```python
from build123d import *

# Parameters (mm, degrees)
SKETCH1_R           = 3.5
BOSS_EXTRUDE1_DEPTH = 2
SKETCH2_R           = 2.75
BOSS_EXTRUDE2_DEPTH = 50.5
SKETCH3_R           = 3.25
BOSS_EXTRUDE3_DEPTH = 1
FILLET1_R           = 1.5
FILLET2_R           = 0.35
FILLET3_R           = 0.2


with BuildPart() as part:
    # Sketch1 → Boss-Extrude1 (new body)
    with BuildSketch(Plane(origin=(0, 0, 0), x_dir=(0, 0, -1), z_dir=(1, 0, 0))):
        Circle(SKETCH1_R)
    extrude(amount=BOSS_EXTRUDE1_DEPTH)

    # Sketch2 → Boss-Extrude2 (add)
    with BuildSketch(Plane(origin=(2, 0, 0), x_dir=(0, 0, -1), z_dir=(1, 0, 0))):
        Circle(SKETCH2_R)
    extrude(amount=BOSS_EXTRUDE2_DEPTH)

    # Sketch3 → Boss-Extrude3 (add)
    with BuildSketch(Plane(origin=(52.5, 0, 0), x_dir=(0, 0, -1), z_dir=(1, 0, 0))):
        Circle(SKETCH3_R)
    extrude(amount=BOSS_EXTRUDE3_DEPTH)

    # Fillet1
    fillet1_edges = [part.edges().sort_by_distance(p)[0] for p in [
        (0, 0, 3.5),
    ]]
    fillet(fillet1_edges, radius=FILLET1_R)

    # Fillet2
    fillet2_edges = [part.edges().sort_by_distance(p)[0] for p in [
        (52.5, 0, 3.25),
    ]]
    fillet(fillet2_edges, radius=FILLET2_R)

    # Fillet3
    fillet3_edges = [part.edges().sort_by_distance(p)[0] for p in [
        (53.5, 0, 3.25),
    ]]
    fillet(fillet3_edges, radius=FILLET3_R)


solid = part.part
```
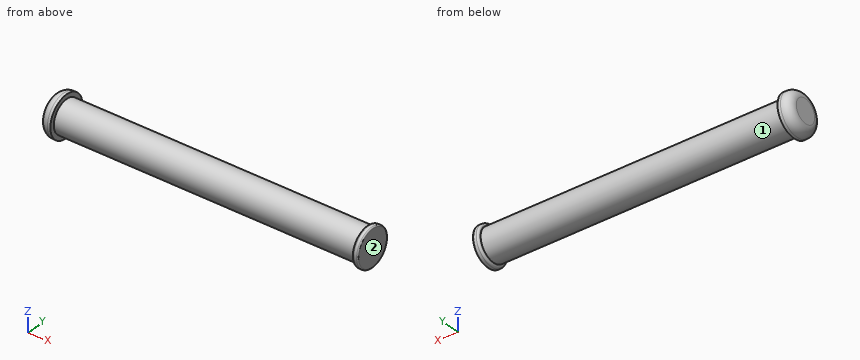
Geometry: final body of the model. Coordinates: model frame, mm. Face numbers are marked on the shaded views. Coordinates: 2 decimals unless noted, no trailing zeros. Order: outer loops, then holes, each group sorted by start corner. A loop starts at its lowest first (then second) coordinate and runs counter-clockwise, first axis right, second up.
Item 1: Draft query along X for the marked faces 1 and 2. Return one class per face: released by +X, released by -X, zero draft, split by the parting line, or undercut.
Answer:
face 1: undercut
face 2: released by +X
Item 2: Material intervals for line 1 along X through (y, z) = (-1.5, 1.5); line 2 along X through (y, z) = (-1, 3); line 3 along Z through (x, y) = (34, 0.25), sorted ascending.
Answer:
line 1: x = 0 to 53.5
line 2: x = 0.55 to 2, 52.62 to 53.47
line 3: z = -2.74 to 2.74
Item 3: Section query C-C (x = 47.5). Output: boundary loops of the cut face in (y, z), then the cut area to 3 significant figures.
Answer:
outline: circle Ø5.5 at (0, 0)
area: 23.8 mm2
Item 4: Contact query for flat-ended pins moving along their axis: P1, Ø4, axis at x = 31, y = 1, coming from the -Z side; P2, Ø1.5, axis at x = 44, z = -1.5, coming from the +Y side. Output: stop coordinate, or through.
Answer:
P1: stops at z = -2.75
P2: stops at y = 2.65
Item 5: Section query A-A (z = 0). Output: boundary loops of the cut face in (x, y), then the cut area to 3 significant figures.
Answer:
outline: (0, -2) arc R1.5 ccw to (1.5, -3.5) - (2, -3.5) - (2, -2.75) - (52.5, -2.75) - (52.5, -2.9) arc R0.35 ccw to (52.85, -3.25) - (53.3, -3.25) arc R0.2 ccw to (53.5, -3.05) - (53.5, 3.05) arc R0.2 ccw to (53.3, 3.25) - (52.85, 3.25) arc R0.35 ccw to (52.5, 2.9) - (52.5, 2.75) - (2, 2.75) - (2, 3.5) - (1.5, 3.5) arc R1.5 ccw to (0, 2) - close
area: 297 mm2
